```python
from build123d import *

# Parameters (mm, degrees)
BOX197_W                                          = 9.8
BOX197_H                                          = 3.4
BOX197_DEPTH                                      = 9.4
CHAMFER218_SIZE                                   = 2.5
CYLINDER692_R                                     = 3
CYLINDER692_DEPTH                                 = 138
CYLINDER688_R                                     = 4.7
CYLINDER688_DEPTH                                 = 3
CYLINDER689_R                                     = 3.2
CYLINDER689_DEPTH                                 = 8
CYLINDER687_R                                     = 4.7
CYLINDER687_DEPTH                                 = 3
CYLINDER686_R                                     = 6
CYLINDER686_DEPTH                                 = 5.5
FUSION088026007031024007017_PLACEMENT_ANGLE       = 180
BOX250_W                                          = 12.8
BOX250_H                                          = 3.6
BOX250_DEPTH                                      = 12.4
CHAMFER228009_SIZE                                = 3
BOX251_W                                          = 12.8
BOX251_H                                          = 3.6
BOX251_DEPTH                                      = 12.4
CHAMFER228008_SIZE                                = 3
CYLINDER685_R                                     = 12
CYLINDER685_DEPTH                                 = 16
CYLINDER690_R                                     = 4.6
CYLINDER690_DEPTH                                 = 3
CYLINDER691_R                                     = 4.6
CYLINDER691_DEPTH                                 = 3
BOX198_W                                          = 9.8
BOX198_H                                          = 3.4
BOX198_DEPTH                                      = 9.4
CHAMFER219_SIZE                                   = 2.5
FUSION088026007031024007008004058_PLACEMENT_ANGLE = 180


with BuildPart() as chamfer218:
    # Box197 → Box197 (new body)
    with BuildSketch(Plane(origin=(2.4, 22.8, 2.8), x_dir=(1, 0, 0), z_dir=(0, 0, 1))):
        with Locations((4.9, 1.7)):
            Rectangle(BOX197_W, BOX197_H)
    extrude(amount=BOX197_DEPTH)

    # Chamfer218
    chamfer218_edges = [chamfer218.edges().sort_by_distance(p)[0] for p in [
        (2.4, 24.5, 12.2),
        (2.4, 24.5, 2.8),
        (12.2, 24.5, 12.2),
        (12.2, 24.5, 2.8),
    ]]
    chamfer(chamfer218_edges, length=CHAMFER218_SIZE)


with BuildPart() as chamfer218_1:
    # Chamfer218 placement: moved
    add(chamfer218.part.moved(Location((-7.5, 33.5, -7.5))))


with BuildPart() as cylinder692:
    # Cylinder692 → Cylinder692 (new body)
    with BuildSketch(Plane(origin=(0, 24, 0), x_dir=(1, 0, 0), z_dir=(0, 1, 0))):
        Circle(CYLINDER692_R)
    extrude(amount=CYLINDER692_DEPTH)


with BuildPart() as cylinder688:
    # Cylinder688 → Cylinder688 (new body)
    with BuildSketch(Plane(origin=(26.5, 52, 7.5), x_dir=(0, 0, -1), z_dir=(1, 0, 0))):
        Circle(CYLINDER688_R)
    extrude(amount=CYLINDER688_DEPTH)


with BuildPart() as cylinder689:
    # Cylinder689 → Cylinder689 (new body)
    with BuildSketch(Plane(origin=(21.5, 52, 7.5), x_dir=(0, 0, -1), z_dir=(1, 0, 0))):
        Circle(CYLINDER689_R)
    extrude(amount=CYLINDER689_DEPTH)


with BuildPart() as cylinder687:
    # Cylinder687 → Cylinder687 (new body)
    with BuildSketch(Plane(origin=(21.5, 52, 7.5), x_dir=(0, 0, -1), z_dir=(1, 0, 0))):
        Circle(CYLINDER687_R)
    extrude(amount=CYLINDER687_DEPTH)


with BuildPart() as pinion_bearings_carving003:
    # Cylinder686 → Cylinder686 (new body)
    with BuildSketch(Plane(origin=(16, 52, 7.5), x_dir=(0, 0, -1), z_dir=(1, 0, 0))):
        Circle(CYLINDER686_R)
    extrude(amount=CYLINDER686_DEPTH)

    # Fusion088026007031024007017: union Cylinder688, Cylinder689, Cylinder687
    add(cylinder688.part)
    add(cylinder689.part)
    add(cylinder687.part)


with BuildPart() as pinion_bearings_carving003_1:
    # Fusion088026007031024007017 placement: moved
    add(pinion_bearings_carving003.part.moved(Location((7.5, 41, 7.5))).rotate(Axis((7.5, 41, 7.5), (0, 1, 0)), FUSION088026007031024007017_PLACEMENT_ANGLE))


with BuildPart() as chamfer228009:
    # Box250 → Box250 (new body)
    with BuildSketch(Plane(origin=(1.1, 21.9, 1.3), x_dir=(1, 0, 0), z_dir=(0, 0, 1))):
        with Locations((6.4, 1.8)):
            Rectangle(BOX250_W, BOX250_H)
    extrude(amount=BOX250_DEPTH)

    # Chamfer228009
    chamfer228009_edges = [chamfer228009.edges().sort_by_distance(p)[0] for p in [
        (1.1, 23.7, 13.7),
        (1.1, 23.7, 1.3),
        (13.9, 23.7, 13.7),
        (13.9, 23.7, 1.3),
    ]]
    chamfer(chamfer228009_edges, length=CHAMFER228009_SIZE)


with BuildPart() as chamfer228009_1:
    # Chamfer228009 placement: moved
    add(chamfer228009.part.moved(Location((-7.5, 59.5, -7.5))))


with BuildPart() as chamfer228008:
    # Box251 → Box251 (new body)
    with BuildSketch(Plane(origin=(1.1, 21.5, 1.3), x_dir=(1, 0, 0), z_dir=(0, 0, 1))):
        with Locations((6.4, 1.8)):
            Rectangle(BOX251_W, BOX251_H)
    extrude(amount=BOX251_DEPTH)

    # Chamfer228008
    chamfer228008_edges = [chamfer228008.edges().sort_by_distance(p)[0] for p in [
        (1.1, 23.3, 13.7),
        (1.1, 23.3, 1.3),
        (13.9, 23.3, 13.7),
        (13.9, 23.3, 1.3),
    ]]
    chamfer(chamfer228008_edges, length=CHAMFER228008_SIZE)


with BuildPart() as chamfer228008_1:
    # Chamfer228008 placement: moved
    add(chamfer228008.part.moved(Location((-7.5, 79.5, -7.5))))


with BuildPart() as cylinder685:
    # Cylinder685 → Cylinder685 (new body)
    with BuildSketch(Plane(origin=(0, 85, 0), x_dir=(1, 0, 0), z_dir=(0, 1, 0))):
        Circle(CYLINDER685_R)
    extrude(amount=CYLINDER685_DEPTH)


with BuildPart() as cylinder690:
    # Cylinder690 → Cylinder690 (new body)
    with BuildSketch(Plane(origin=(0, 24, 0), x_dir=(1, 0, 0), z_dir=(0, 1, 0))):
        Circle(CYLINDER690_R)
    extrude(amount=CYLINDER690_DEPTH)


with BuildPart() as cylinder691:
    # Cylinder691 → Cylinder691 (new body)
    with BuildSketch(Plane(origin=(0, 159, 0), x_dir=(1, 0, 0), z_dir=(0, 1, 0))):
        Circle(CYLINDER691_R)
    extrude(amount=CYLINDER691_DEPTH)


with BuildPart() as inner_carving_rear:
    # Box198 → Box198 (new body)
    with BuildSketch(Plane(origin=(2.4, 22.8, 2.8), x_dir=(1, 0, 0), z_dir=(0, 0, 1))):
        with Locations((4.9, 1.7)):
            Rectangle(BOX198_W, BOX198_H)
    extrude(amount=BOX198_DEPTH)

    # Chamfer219
    chamfer219_edges = [inner_carving_rear.edges().sort_by_distance(p)[0] for p in [
        (2.4, 24.5, 12.2),
        (2.4, 24.5, 2.8),
        (12.2, 24.5, 12.2),
        (12.2, 24.5, 2.8),
    ]]
    chamfer(chamfer219_edges, length=CHAMFER219_SIZE)


with BuildPart() as inner_carving_rear_1:
    # Chamfer219 placement: moved
    add(inner_carving_rear.part.moved(Location((-7.5, 103.5, -7.5))))

    # Fusion088026007031024007008004058: union Chamfer218, Cylinder692, pinion-bearings-carving003, Chamfer228009, Chamfer228008, Cylinder685, Cylinder690, Cylinder691
    add(chamfer218_1.part)
    add(cylinder692.part)
    add(pinion_bearings_carving003_1.part)
    add(chamfer228009_1.part)
    add(chamfer228008_1.part)
    add(cylinder685.part)
    add(cylinder690.part)
    add(cylinder691.part)


with BuildPart() as inner_carving_rear_2:
    # Fusion088026007031024007008004058 placement: moved
    add(inner_carving_rear_1.part.moved(Location((75, -93, 46))).rotate(Axis((75, -93, 46), (0, 1, 0)), FUSION088026007031024007008004058_PLACEMENT_ANGLE))


solid = inner_carving_rear_2.part
```
The model under review builds one solid part; all positions refer to its coordinate system, in mm. A direction names the side the tool comes from. Round coordinates to 2 decimals unless told otherwise and drop trailing zeros. Loops run counter-clockwise (first coordinate to the right, second up) from the corner with the lowest first, then second, coordinate; pieces in that order, holes last.
Item 1: For faces 1 (the face through (70.3, 35, 46)), 2 (the face through (77.45, 36.7, 43.98)), 3 (the face through (75, 10, 52.2)), 4 (the face through (70, 8, 41)), list the 3-axis set-ups (+Z, -Z, +X, -X, +Y, -Y) from which the entire face can be reached by the end or side of a thin tool; tool diameter is ignored.
Determined:
face 1: +Z, -Z, -X, +Y
face 2: none
face 3: +Z, +X, -X, +Y
face 4: +Y
Item 2: Mouldability with a two-part tool opening along Y and no side actions: class faces 5 (the face through (70, -8, 41)), 6 (the face through (71.6, 35, 42.5)), 7 (the face through (74, -66, 43)) as released by +Y, released by -Y, zero draft, split by the parting line, or undercut.
Determined:
face 5: released by -Y
face 6: zero draft
face 7: undercut
Item 3: Take a section at C-C (x = 84). Write out the cut boundary in (y, z), then the cut area to 3 significant figures.
Determined:
outline: (-8, 38.06) - (8, 38.06) - (8, 53.94) - (-8, 53.94) - close
area: 254 mm2
Item 4: For line 1 (Y direction, x = 80, z = 44); line 2 (Y direction, x = 67, z = 44.25); line 3 (Y direction, x = 70.5, z = 42.25), list the stretches that pass through material, from the lowest coordinate up.
Determined:
line 1: y = -36.7 to -33.3, -11.6 to 11.6, 33.3 to 36.7
line 2: y = -8 to 8
line 3: y = -11.6 to 11.6
Item 5: Take a section at A-A (y = 0). Write out the cut boundary in (x, z), then the cut area to 3 significant figures.
Determined:
outline: (85.39, 40) - (89, 40) - (89, 41.3) - (92, 41.3) - (92, 42.8) - (94, 42.8) - (94, 41.3) - (97, 41.3) - (97, 50.7) - (94, 50.7) - (94, 49.2) - (92, 49.2) - (92, 50.7) - (89, 50.7) - (89, 52) - (85.39, 52) arc R12 ccw (long way) to start
area: 552 mm2
Item 6: Clearance check with flat-ended pins moving along their axes: pin 1 Ø12 at (y, z) = (34.5, 39.5) entering from +X; pin 2 Ø1.5 at (x, y) = (72, 30.5) entering from -Z; pin 3 Ø3.5 at (x, y) = (74.5, 35) entering from +Z. State where each tip first meets the part, or that it passes through.
Determined:
pin 1: stops at x = 80.1
pin 2: stops at z = 44.02
pin 3: stops at z = 50.7
Item 7: Take a section at D-D (y = 14). Write out the cut boundary in (x, z).
Determined:
outline: circle Ø6 at (75, 46)
Item 8: Take a section at B-B (z = 38.5). Write out the cut boundary in (x, y), then the cut area to 3 significant figures.
Determined:
outline: (65.63, -8) - (84.37, -8) - (84.37, 8) - (65.63, 8) - close
area: 300 mm2
